CAD build for the part. Positions are in the model's coordinates, mm. Coordinates: 2 decimals unless noted, no trailing zeros. Loops run counter-clockwise (first coordinate to the right, second up) from the corner with the lowest first, then second, coordinate; pieces in that order, holes last. Notation, with made-up numbers: (77.5, 18) -> (107.5, 18) arc R33 cw to (107.5, 51) -> close; hole circle Ø7 at (-4.5, -3.75). An arc over 180 degrees is marked (long way). Write each question's results on one line, items separated by ' | '.
Autodesk Inventor part; units mm, degrees
ref_plane "YZ Plane" through (0, 0, 0) normal (1, 0, 0) x (0, 1, 0)
ref_plane "XZ Plane" through (0, 0, 0) normal (0, 1, 0) x (-1, 0, 0)
ref_plane "XY Plane" through (0, 0, 0) normal (0, 0, 1) x (1, 0, 0)
sketch "Sketch1" plane through (0, 0, 0) normal (0, 0, 1) x (1, 0, 0)
  line L0 (-9.3881, 16.2606) -> (9.3868, 16.2606)
  line L1 (18.7092, 0.25) -> (18.7092, 0.25)
  line L2 (18.7762, 0) -> (9.3868, 16.2606)
  line L3 (18.7762, 0) -> (9.3868, -16.2606)
  line L4 (-9.3881, -16.2606) -> (9.3868, -16.2606)
  line L5 (-18.7762, 0) -> (-9.3881, -16.2606)
  line L6 (-18.7762, 0) -> (-9.3881, 16.2606)
  circle A0 centre (16, 0) radius 2
  circle A1 centre (8, 13.8564) radius 2
  circle A2 centre (-8, 13.8564) radius 2
  circle A3 centre (-16, 0) radius 2
  circle A4 centre (8, -13.8564) radius 2
  circle A5 centre (-8, -13.8564) radius 2
  circle A6 centre (0, 0) radius 6.35
  circle A7 centre (-0.0003, -14.1904) radius 1.8542
  circle A8 centre (0.001, 14.1866) radius 1.8542
  circle A9 centre (12.2905, 7.0829) radius 1.8542
  circle A10 centre (12.2905, -7.0852) radius 1.8542
  circle A11 centre (-12.2865, -7.0924) radius 1.8542
  circle A12 centre (-12.2865, 7.0829) radius 1.8542
  dimension "d3" = 12.7
  dimension "d4" = 3.7084
  dimension "d5" = 3.7084
  dimension "d6" = 3.7084
  dimension "d7" = 3.7084
  dimension "d8" = 3.7084
  dimension "d9" = 3.7084
extrude "Extrusion1" add sketch "Sketch1" along normal blind 2.9718
properties part number "90d Spacer"
1) Slice it at A-A (x = 0). Write the cut outline in (y, z), then the cut area to 3 significant figures.
Outcome:
outline: (-16.26, 0) -> (-16.04, 0) -> (-16.04, 2.97) -> (-16.26, 2.97) -> close; (-12.34, 0) -> (-6.35, 0) -> (-6.35, 2.97) -> (-12.34, 2.97) -> close; (6.35, 0) -> (12.33, 0) -> (12.33, 2.97) -> (6.35, 2.97) -> close; (16.04, 0) -> (16.26, 0) -> (16.26, 2.97) -> (16.04, 2.97) -> close | area: 36.9 mm^2
2) Slice it at D-D (z = 1.1). Count the separate pieces of the cut face and the enclosed holes in it, then the cut area to 3 significant figures.
Outcome:
separate pieces: 1 | enclosed holes: 13 | area: 649 mm^2
3) Two-plate mould, pull along X, no slides. Class faces 1 (the flat face through (14.147, 8.016, 1.465)), 2 (the flat face through (0, -16.261, 1)), 3 (the cylindrical face through (-11.43, -5.45, 1.47)): pulls with the +X half, pulls with the -X half, needs draft (parallel to the pull), parting line crosses it, or undercut.
Outcome:
face 1: pulls with the +X half | face 2: needs draft | face 3: undercut
4) Slice it at C-C (y = -7.5). Write the cut outline in (x, z).
Outcome:
outline: (-14.45, 0) -> (-14.1, 0) -> (-14.1, 2.97) -> (-14.45, 2.97) -> close; (-10.48, 0) -> (10.48, 0) -> (10.48, 2.97) -> (-10.48, 2.97) -> close; (14.1, 0) -> (14.45, 0) -> (14.45, 2.97) -> (14.1, 2.97) -> close
5) Slice it at B-B (x = 8). Write the cut outline in (y, z), then the cut area to 3 significant figures.
Outcome:
outline: (-16.26, 0) -> (-15.86, 0) -> (-15.86, 2.97) -> (-16.26, 2.97) -> close; (-11.86, 0) -> (11.86, 0) -> (11.86, 2.97) -> (-11.86, 2.97) -> close; (15.86, 0) -> (16.26, 0) -> (16.26, 2.97) -> (15.86, 2.97) -> close | area: 72.9 mm^2
6) Drill centre lines: L1, parallel to Y at x = -8, z = 2.1; L2, parallel to X at y = -1, z = 2.3; L3, parallel to Y at x = 8.5, z = 1.5. Where is each one in solid material? Low to high. Write a range as from..to.
Outcome:
L1: y = -16.26..-15.86, -11.86..11.86, 15.86..16.26 | L2: x = -18.2..-17.73, -14.27..-6.27, 6.27..14.27, 17.73..18.2 | L3: y = -16.26..-15.79, -11.92..11.92, 15.79..16.26
7) Pin check, flat tip, straight feed: pin 1 (1 mm diameter, centred on y = -7, z = 2.5, fed in from -X). Stop position of the tip, or through.
Outcome:
pin 1: stops at x = -15.02
